```python
from build123d import *

# Parameters (mm, degrees)
F0_W     = 146.409408
F0_H     = 112.187884
F0_W_2   = 134.296582
F0_H_2   = 96.886568
F1_DEPTH = 76.2
F2_W     = 71.00363
F2_H     = 39.288416
F3_DEPTH = 112.188885
F4_R     = 9.066192
F5_DEPTH = 146.410407


with BuildPart() as f1:
    # F0 (on Top) → F1 (new body)
    with BuildSketch(Plane.XY):
        Rectangle(F0_W, F0_H)
        Rectangle(F0_W_2, F0_H_2, mode=Mode.SUBTRACT)
    extrude(amount=F1_DEPTH)

    # F2 (on face) → F3 (cut, through all)
    with BuildSketch(Plane.XZ.offset(56.093942)):
        with Locations((0, 95.844208)):
            Rectangle(F2_W, F2_H)
        with Locations((0, 56.555792)):
            Rectangle(F2_W, F2_H)
    extrude(amount=-F3_DEPTH, mode=Mode.SUBTRACT)

    # F4 (on face) → F5 (cut, through all)
    with BuildSketch(Plane.YZ.offset(73.204704)):
        with Locations((0, 38.1)):
            Circle(F4_R)
    extrude(amount=-F5_DEPTH, mode=Mode.SUBTRACT)


solid = f1.part
```
Design review of the part built by this model. Coordinates are the model's own, in mm. A direction names the side the tool comes from. Coordinates: 2 decimals unless noted, no trailing zeros. Order: outer loops, then holes, each group sorted by start corner. A loop starts at its lowest first (then second) coordinate and runs counter-clockwise, first axis right, second up. Notation, with made-up numbers: M 29.25,10.5 L 68.25,10.5 A29 cw 68.25,44.5 Z; hole C 13,85 d6. An arc over 180 degrees is marked long. Answer as a JSON object with one key per item and string values. Group by question number.
1) Add section B-B, the plane y = 39. Write out the cut boundary in (x, z).
2) Mouldability with a two-part tool opening along Y and no side actions: class faces 4 (the flat face through (-1, 56.094, 29)), 5 (the flat face through (35.502, -52, 56)), 6 (the flat face through (-67.148, -11, 38)) as pulls with the +Y half, pulls with the -Y half, needs draft (parallel to the pull), parting line crosses it, or undercut.
3) Add section D-D, the plane y = 0. Write out the cut boundary in (x, z), then the cut area to 3 significant figures.
4) Add section C-C, the plane z = 50.5. Write out the cut boundary in (x, y).
5) Add section A-A, the plane x = 1.5. Write out the cut boundary in (y, z), then the cut area to 3 significant figures.
6) Wall thickness on L1, parallel to Z at x = 71, y = 0; L2, parallel to X at y = 1, z = 64; L3, parallel to Y at x = 57.5, z = 25: over which ranges is each line inside the solid? List them lowest first.
7) Tool access review of faces 1 (the flat face through (-35.502, 52, 57)), 2 (the cylindrical face through (70.219, 4.874, 45.745)), 3 (the flat face through (-1, -48.443, 29)): name each direction out of +Z, -Z, +X, -X, +Y, -Y from which nothing blocks a thin tool from reaching the whole face with its end or side.
8) For pin 1 (2.5 mm diameter, centred on x = -11, y = 53.5, fed in from +Z); pin 2 (23 mm diameter, centred on x = -32, z = 55.5, fed in from +Y), all flat-tipped, find the tip position at first contact; note any pin that passes through.
Computed values:
{
 "1": {"outline": "M -73.2,0 L -67.15,0 L -67.15,76.2 L -73.2,76.2 Z; M 67.15,0 L 73.2,0 L 73.2,76.2 L 67.15,76.2 Z"},
 "2": {"face 4": "pulls with the +Y half", "face 5": "needs draft", "face 6": "undercut"},
 "3": {"outline": "M -73.2,0 L -67.15,0 L -67.15,29.03 L -73.2,29.03 Z; M -73.2,47.17 L -67.15,47.17 L -67.15,76.2 L -73.2,76.2 Z; M 67.15,0 L 73.2,0 L 73.2,29.03 L 67.15,29.03 Z; M 67.15,47.17 L 73.2,47.17 L 73.2,76.2 L 67.15,76.2 Z", "area": "703 mm^2"},
 "4": {"outline": "M -73.2,-56.09 L -35.5,-56.09 L -35.5,-48.44 L -67.15,-48.44 L -67.15,48.44 L -35.5,48.44 L -35.5,56.09 L -73.2,56.09 Z; M 35.5,-56.09 L 73.2,-56.09 L 73.2,56.09 L 35.5,56.09 L 35.5,48.44 L 67.15,48.44 L 67.15,-48.44 L 35.5,-48.44 Z"},
 "5": {"outline": "M -56.09,0 L -48.44,0 L -48.44,36.91 L -56.09,36.91 Z; M 48.44,0 L 56.09,0 L 56.09,36.91 L 48.44,36.91 Z", "area": "565 mm^2"},
 "6": {"L1": "z = 0 to 29.03, 47.17 to 76.2", "L2": "x = -73.2 to -67.15, 67.15 to 73.2", "L3": "y = -56.09 to -48.44, 48.44 to 56.09"},
 "7": {"face 1": "+Z, +Y, -Y", "face 2": "+X, -X", "face 3": "+Z, -Z"},
 "8": {"pin 1": "stops at z = 36.91", "pin 2": "stops at y = 56.09"}
}
